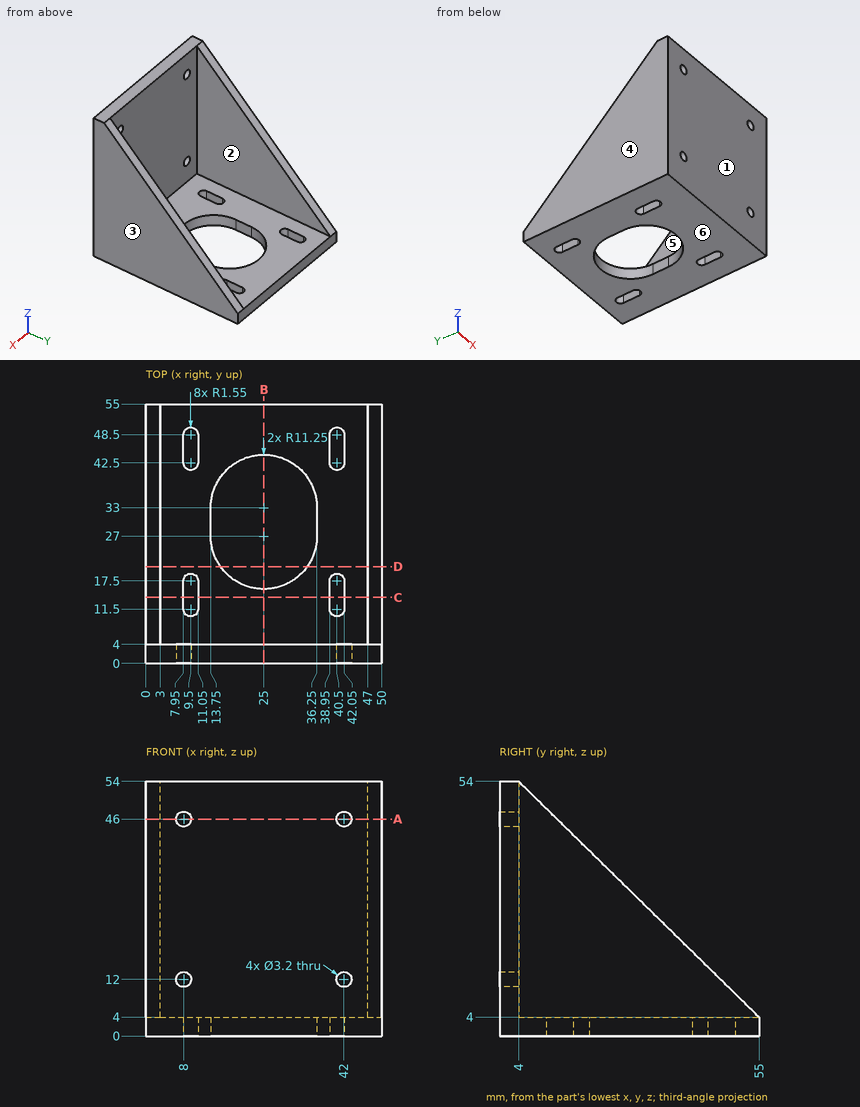
Check sheet for the drawn part. Datum: minimum x, y, z corner. Units: mm. A direction names the side the tool comes from. Give positions to 0.01 mm unless a question says otherwise; leave off trailing zeros. Write each loop counter-clockwise with the first axis right and the second up, starting at its lowest first coordinate (ties: lowest second). Pieces come first, ordered by that corner, then holes. Notation, with made-up numbers: M -25,77 L -15,77 A34 ccw -15,110 Z; hole C 45.5,85 d7. An arc over 180 degrees is marked long. Write item = value, one per line.
(1) Sectioned sample at A-A (z = 46). Record the cut outline in (x, y), then the cut area to 3 significant figures.
Found:
outline = M 0,0 L 6.4,0 L 6.4,4 L 3,4 L 3,12.16 L 0,12.16 Z; M 9.6,0 L 40.4,0 L 40.4,4 L 9.6,4 Z; M 43.6,0 L 50,0 L 50,12.16 L 47,12.16 L 47,4 L 43.6,4 Z
area = 223 mm2
(2) Sectioned sample at C-C (y = 14). Record the cut outline in (x, z), then the cut area to 3 significant figures.
Found:
outline = M 0,0 L 7.95,0 L 7.95,4 L 3,4 L 3,44.2 L 0,44.2 Z; M 11.05,0 L 38.95,0 L 38.95,4 L 11.05,4 Z; M 42.05,0 L 50,0 L 50,44.2 L 47,44.2 L 47,4 L 42.05,4 Z
area = 416 mm2
(3) Go/stop test with flat-tipped pins: pin 1 Ø8 at (x, z) = (8, 42) entering from +Y; pin 2 Ø2 at (x, y) = (41, 25) entering from +Z. Record where each tip stops, or that it passes through.
Found:
pin_1 = 4
pin_2 = 4
(4) Sectioned sample at D-D (y = 20.5). Record the cut outline in (x, z).
Found:
outline = M 0,0 L 15.82,0 L 15.82,4 L 3,4 L 3,37.82 L 0,37.82 Z; M 34.18,0 L 50,0 L 50,37.82 L 47,37.82 L 47,4 L 34.18,4 Z
(5) Material ranges on line 1 (X direction, y = 1.8, z = 46); line 2 (X direction, y = 6, z = 39); line 3 (Y direction, x = 38.5, z = 13), recorded low to high.
Found:
line_1 = 0 to 6.4, 9.6 to 40.4, 43.6 to 50
line_2 = 0 to 3, 47 to 50
line_3 = 0 to 4
(6) Access from +Z, -Z, +X, -X, +Y, -Y to the whole of each face (thin tool, end or side, straight path). Record for the marked faces 1 and 2.
Found:
face_1 = +Z, -Z, +X, -X, -Y
face_2 = +Z, +Y
(7) Draft check along X on the marked faces 3, 4, 5 and 6. Enter one of: released by +X, released by -X, zero draft, split by the parting line, or undercut.
Found:
face_3 = released by +X
face_4 = released by -X
face_5 = undercut
face_6 = zero draft
(8) Sectioned sample at B-B (x = 25). Record the cut outline in (y, z).
Found:
outline = M 0,0 L 15.75,0 L 15.75,4 L 4,4 L 4,54 L 0,54 Z; M 44.25,0 L 55,0 L 55,4 L 44.25,4 Z
